```python
from build123d import *

# Parameters (mm, degrees)
SKETCH1_R             = 7
BOSS_EXTRUDE1_DEPTH   = 40.99
SKETCH2_W             = 14.337226175
SKETCH2_H             = 3.81556612
BOSS_EXTRUDE2_DEPTH   = 3
SKETCH2_W_2           = 14.616397067
BOSS_EXTRUDE2_2_DEPTH = 3
SKETCH3_W             = 14.616397067
SKETCH3_H             = 3.81556612
SKETCH3_W_2           = 14.337226175
BOSS_EXTRUDE3_DEPTH   = 10


with BuildPart() as part:
    # Sketch1 → Boss-Extrude1 (new body)
    with BuildSketch(Plane(origin=(0, 0, 0), x_dir=(0, 0, -1), z_dir=(1, 0, 0))):
        Circle(SKETCH1_R)
    extrude(amount=BOSS_EXTRUDE1_DEPTH)



with BuildPart() as body_2:
    # Sketch2 → Boss-Extrude2 (new body)
    with BuildSketch(Plane(origin=(0, -5.457447914, -4.383635737), x_dir=(1, 0, 0), z_dir=(0, -0.779635416, -0.626233677))):
        with Locations((7.168613088, 0.421848142)):
            Rectangle(SKETCH2_W, SKETCH2_H)
    extrude(amount=BOSS_EXTRUDE2_DEPTH)


with BuildPart() as body_3:
    # Sketch2 → Boss-Extrude2 2 (new body)
    with BuildSketch(Plane(origin=(0, -5.457447914, -4.383635737), x_dir=(1, 0, 0), z_dir=(0, -0.779635416, -0.626233677))):
        with Locations((33.681801467, 0.421848142)):
            Rectangle(SKETCH2_W_2, SKETCH2_H)
    extrude(amount=BOSS_EXTRUDE2_2_DEPTH)


with BuildPart() as part_1:
    add(part.part)

    add(body_2.part)  # Boss-Extrude3 merges body 2

    add(body_3.part)  # Boss-Extrude3 merges body 3
    # Sketch3 → Boss-Extrude3 (add)
    with BuildSketch(Plane(origin=(0, -5.457447914, -4.383635737), x_dir=(1, 0, 0), z_dir=(0, 0.779635416, 0.626233677))):
        with Locations((33.681801467, -0.421848142)):
            Rectangle(SKETCH3_W, SKETCH3_H)
        with Locations((7.168613088, -0.421848142)):
            Rectangle(SKETCH3_W_2, SKETCH3_H)
    extrude(amount=BOSS_EXTRUDE3_DEPTH)


solid = part_1.part
```
Could you check a few things on this model? Use its own coordinates, in mm. A direction names the side the tool comes from. Round coordinates to 2 decimals unless told otherwise and drop trailing zeros. Loops run counter-clockwise (first coordinate to the right, second up) from the corner with the lowest first, then second, coordinate; pieces in that order, holes last. Notation, with made-up numbers: (-12, 25.25) - (-6, 25.25) arc R19 cw to (-6, 49.25) - close; hole circle Ø10 at (28, -32.5). An arc over 180 degrees is marked (long way). Answer in a Markdown table with one row per item. Add a question column.
(1) If we section it at C-C (x = 24): Please give me the cut outline in (y, z).
(2) I'm going to push a flat-ended pin straight in: pin 1 (8 mm diameter, centred on x = 14.5, y = -2.5, fed in from -Z). Where does the tip first touch, or does it pass through?
(3) If we mould it in two halves opening along Y, with no side actions, what happens to faces 1 (the face through (0, -1, 0)), 2 (the face through (33.58, -5.62, -6.42)), 3 (the face through (7.07, -7.95, -3.4))? For each: pulls with the +Y half, pulls with the -Y half, needs draft (parallel to the pull), parting line crosses it, or undercut.
(4) If we section it at B-B (z = -5): Please give me the cut outline in (x, y).
(5) If we section it at D-D (y = 0): Please give me the cut outline in (x, z), plus the area to 3 significant figures.
(6) I need wall thicknesses on line 1 along Z through (x, y) = (27, 0.25); line 2 along Z through (x, y) = (8.5, 3); line 3 along Y through (x, z) = (2, -1). Which ranges of each line are inside material? Lowest first, please.
(7) For faces 4 (the face through (26.374, -7, -5)), 5 (the face through (7.068, -5.651, -6.445)), 6 (the face through (33.58, -8.08, -5.91)), which set-ups out of +Z, -Z, +X, -X, +Y, -Y let a thin tool reach every point of the face, with its end or its side?
(8) If we section it at A-A (y = -7.5): Please give me the cut outline in (x, z).
Model answer:
| question | item | result |
|---|---|---|
| 1 | outline | circle Ø14 at (0, 0) |
| 2 | pin 1 | stops at z = -7.12 |
| 3 | face 1 | needs draft |
| 3 | face 2 | undercut |
| 3 | face 3 | pulls with the -Y half |
| 4 | outline | (0, -8.81) - (14.34, -8.81) - (14.34, -4.9) - (26.37, -4.9) - (26.37, -8.81) - (40.99, -8.81) - (40.99, 4.9) - (0, 4.9) - close |
| 5 | outline | (0, -7) - (40.99, -7) - (40.99, 7) - (0, 7) - close |
| 5 | area | 574 mm² |
| 6 | line 1 | z = -7 to 7 |
| 6 | line 2 | z = -6.32 to 6.32 |
| 6 | line 3 | y = -6.93 to 6.93 |
| 7 | face 4 | -Z, -Y |
| 7 | face 5 | -Z, +X, -X |
| 7 | face 6 | -Z, +X, -X, -Y |
| 8 | outline | (0, -6.63) - (14.34, -6.63) - (14.34, -3.04) - (0, -3.04) - close; (26.37, -6.63) - (40.99, -6.63) - (40.99, -3.04) - (26.37, -3.04) - close |
